Input: part model. Units: mm. Frame: model coordinates. A direction names the side the tool comes from. Give positions to 0.01 mm unless a question says otherwise; leave off trailing zeros. Order: outer loops, then holes, each group sorted by start corner. A loop starts at its lowest first (then second) coordinate and runs counter-clockwise, first axis right, second up. Notation, with made-up numbers: M -24.75,-1.5 L 17.25,-1.5 A16 cw 17.25,14.5 Z; hole C 65,24 d7. An arc over 180 degrees is marked long. Use a Markdown table: item, result.
from build123d import *

# Parameters (mm, degrees)
F1_DEPTH  = 63.5
F2_DEPTH  = 25.4
F4_E5_0_W = 28.3572662234
F4_E5_0_H = 50.8
F5_DEPTH  = 19.05
F6_DEPTH  = 7.9375
F7_R      = 5.08


with BuildPart() as f1:
    # F0 (on Front) → F1 (new body, symmetric)
    with BuildSketch(Plane.XZ):
        Polygon((-41.275, 9.525), (-41.275, -9.525), (41.275, -9.525), (41.275, 9.525), (22.225, 9.525), align=None)
    extrude(amount=F1_DEPTH, both=True)

    # F0 (on Front) → F2 (join, symmetric)
    with BuildSketch(Plane.XZ):
        with BuildLine():
            Line((22.225, 9.525), (41.275, 9.525))
            Line((41.275, 9.525), (41.275, 27.0002))
            ThreePointArc((41.275, 27.0002), (45.9246798487, 38.2255201513), (57.15, 42.8752))
            Line((57.15, 42.8752), (60.325, 42.8752))
            Line((60.325, 42.8752), (60.325, 61.9252))
            Line((60.325, 61.9252), (57.15, 61.9252))
            add(Edge.make_bspline(
                [(50.2742596594, 61.2416926627), (52.505084267, 61.4836028987), (54.7963675205, 61.7116076427), (57.15, 61.9252)],
                knots=[108.25411783, 108.25411783, 108.25411783, 108.25411783, 111.5045361635, 111.5045361635, 111.5045361635, 111.5045361635], degree=3))
            ThreePointArc((50.2742596594, 61.2416926627), (30.1324977432, 49.1318559887), (22.225, 27.0002))
            Line((22.225, 27.0002), (22.225, 9.525))
        make_face()
    extrude(amount=F2_DEPTH, both=True)

    # F0 (on Front) → F3 (revolve)
    with BuildSketch(Plane.XZ):
        Polygon((85.5072662234, 66.675), (85.6886142667, 42.8752), (85.725, 38.1), (111.125, 38.1), (111.125, 66.675), align=None)
    revolve(axis=Axis((85.6161331117, 0, 52.3875), (-0.0076195085, 0, 0.9999709711)))

    # F4_E5_0 (on explicit) → F5 (join)
    with BuildSketch(Plane(origin=(57.15, 25.4, 61.9252), x_dir=(1, 0, 0), z_dir=(0, 0, -1))):
        with Locations((14.1786331117, 25.4)):
            Rectangle(F4_E5_0_W, F4_E5_0_H)
    extrude(amount=F5_DEPTH)

    # F0 (on Front) → F6 (join, symmetric)
    with BuildSketch(Plane.XZ):
        with BuildLine():
            add(Edge.make_bspline(
                [(-41.275, 9.525), (-31.2587030045, 29.7042218625), (-24.022623126, 53.1849514965), (50.2742596594, 61.2416926627)],
                knots=[0, 0, 0, 0, 108.25411783, 108.25411783, 108.25411783, 108.25411783], degree=3))
            Line((-41.275, 9.525), (22.225, 9.525))
            Line((22.225, 9.525), (22.225, 27.0002))
            ThreePointArc((22.225, 27.0002), (30.1324977432, 49.1318559887), (50.2742596594, 61.2416926627))
        make_face()
    extrude(amount=F6_DEPTH, both=True)

    # F7
    f7_edges = [f1.edges().sort_by_distance(p)[0] for p in [
        (41.275, -63.5, 0),
        (-41.275, -63.5, 0),
        (-41.275, 63.5, 0),
        (41.275, 63.5, 0),
    ]]
    fillet(f7_edges, radius=F7_R)


solid = f1.part
1) Reachability of faces 5 (the face through (-5, 7.938, 30)), 6 (the face through (41.275, -1, 4)), 7 (the face through (87.2, -0.6, 38.1)) from +Z, -Z, +X, -X, +Y, -Y: full face, straight path, thin tool, end or side. Return the list, or none.
Response values:
| item | result |
|---|---|
| face 5 | +Z, -X, +Y |
| face 6 | -Z, +X, +Y, -Y |
| face 7 | -Z, +X |
2) Material intervals for line 1 (Y direction, x = 64, z = 48); line 2 (Z direction, x = 6.5, y = 39) (3 decimals); line 3 (Y direction, x = 3.5, z = 18.5), sorted ascending. Write a range as from..to.
Response values:
| item | result |
|---|---|
| line 1 | y = -25.4..25.4 |
| line 2 | z = -9.525..9.525 |
| line 3 | y = -7.94..7.94 |
3) Mould query, pull axis X, two halves, no side actions, for faces 1 (the face through (60, 2, 42.875)), 2 (the face through (45.8, -0.4, 38.1)), 3 (the face through (1, 35, 9.525)), 4 (the face through (39.75, -62.05, 0.13)). Classes: released by +X, released by -X, zero draft, split by the parting line, or undercut.
Response values:
| item | result |
|---|---|
| face 1 | undercut |
| face 2 | undercut |
| face 3 | zero draft |
| face 4 | released by +X |
4) First-contact query: pin 1 Ø3 at (x, y) = (5.5, 35) entering from +Z (3 decimals); pin 2 Ø12.5 at (x, y) = (66, 3.5) entering from +Z; pin 3 Ø8 at (x, y) = (67, -0.5) entering from -Z; pin 4 Ø8 at (y, z) = (-31, 53.5) entering from -X. Flat tips, straight axial feed; report the tip coordinate or a pass-through.
Response values:
| item | result |
|---|---|
| pin 1 | stops at z = 9.525 |
| pin 2 | stops at z = 66.47 |
| pin 3 | stops at z = 37.75 |
| pin 4 | passes through |
5) Cut plane A-A on y = -54.5. Return loops of the section in (x, z) (3 decimals).
Response values:
| item | result |
|---|---|
| outline | M -41.275,-9.525 L 41.275,-9.525 L 41.275,9.525 L -41.275,9.525 Z |
